```python
from build123d import *

# Parameters (mm, degrees)
SKETCH1_R           = 2.7305
BOSS_EXTRUDE1_DEPTH = 4.6355
SKETCH2_W           = 10.4775
SKETCH2_H           = 9.271
BOSS_EXTRUDE2_DEPTH = 2.54
SKETCH3_W           = 10.4775
SKETCH3_H           = 2.54
SKETCH3_W_2         = 7.8105
SKETCH3_H_2         = 10.4775
BOSS_EXTRUDE3_DEPTH = 7.366
SKETCH4_W           = 3.302
SKETCH4_H           = 6.604
CUT_EXTRUDE1_DEPTH  = 10.4775
FILLET1_R           = 0.762


with BuildPart() as part:
    # Sketch1 → Boss-Extrude1 (new body, symmetric)
    with BuildSketch(Plane(origin=(0, 0, 0), x_dir=(1, 0, 0), z_dir=(0, 1, 0))):
        Polygon((-11.1125, 3.81), (-4.191, 3.81), (-4.191, 9.144), (6.2865, 9.144), (6.2865, -6.6675), (-11.1125, -6.6675), align=None)
        Circle(SKETCH1_R, mode=Mode.SUBTRACT)
    extrude(amount=BOSS_EXTRUDE1_DEPTH, both=True)

    # Sketch2 → Boss-Extrude2 (add)
    with BuildSketch(Plane.ZY.offset(11.1125)):
        with Locations((1.42875, 0)):
            Rectangle(SKETCH2_W, SKETCH2_H)
    extrude(amount=BOSS_EXTRUDE2_DEPTH)

    # Sketch3 → Boss-Extrude3 (add, symmetric)
    with BuildSketch(Plane(origin=(0, 0, 0), x_dir=(1, 0, 0), z_dir=(0, 1, 0))):
        with Locations((1.04775, 7.874)):
            Rectangle(SKETCH3_W, SKETCH3_H)
        with Locations((-9.74725, -1.42875)):
            Rectangle(SKETCH3_W_2, SKETCH3_H_2)
    extrude(amount=BOSS_EXTRUDE3_DEPTH, both=True)

    # Sketch4 → Cut-Extrude1 (cut)
    with BuildSketch(Plane(origin=(0, 0, -3.81), x_dir=(-1, 0, 0), z_dir=(0, 0, -1))):
        with Locations((8.636, 0)):
            Rectangle(SKETCH4_W, SKETCH4_H)
    extrude(amount=-CUT_EXTRUDE1_DEPTH, mode=Mode.SUBTRACT)

    # Fillet1
    fillet1_edges = [part.edges().sort_by_distance(p)[0] for p in [
        (6.2865, 4.6355, 0.03175),
        (-4.191, 0, -3.81),
        (-4.191, 0, -9.144),
        (6.2865, 0, -9.144),
        (6.2865, 0, 6.6675),
        (-5.0165, 4.6355, -3.81),
        (-13.6525, 0, -3.81),
        (-13.6525, 0, 6.6675),
        (-4.191, -4.6355, -5.207),
        (-4.191, 4.6355, -5.207),
        (6.2865, 6.00075, -6.604),
        (-4.191, 6.00075, -6.604),
        (6.2865, -6.00075, -6.604),
        (6.2865, -7.366, -7.874),
        (1.04775, -7.366, -9.144),
        (-4.191, -7.366, -7.874),
        (-4.191, -6.00075, -6.604),
        (1.04775, -7.366, -6.604),
        (6.2865, 7.366, -7.874),
        (1.04775, 7.366, -9.144),
        (-4.191, 7.366, -7.874),
        (1.04775, 7.366, -6.604),
        (0.22225, -4.6355, 6.6675),
        (0.22225, 4.6355, 6.6675),
        (-5.842, 6.00075, 6.6675),
        (-5.842, 6.00075, -3.81),
        (-5.842, -6.00075, 6.6675),
        (-5.842, -7.366, 1.42875),
        (-5.842, -6.00075, -3.81),
        (-9.74725, -7.366, -3.81),
        (-13.6525, -7.366, 1.42875),
        (-9.74725, -7.366, 6.6675),
        (-5.0165, -4.6355, -3.81),
        (-5.842, 7.366, 1.42875),
        (-9.74725, 7.366, -3.81),
        (-13.6525, 7.366, 1.42875),
        (-9.74725, 7.366, 6.6675),
        (6.2865, -4.6355, 0.03175),
    ]]
    fillet(fillet1_edges, radius=FILLET1_R)


solid = part.part
```
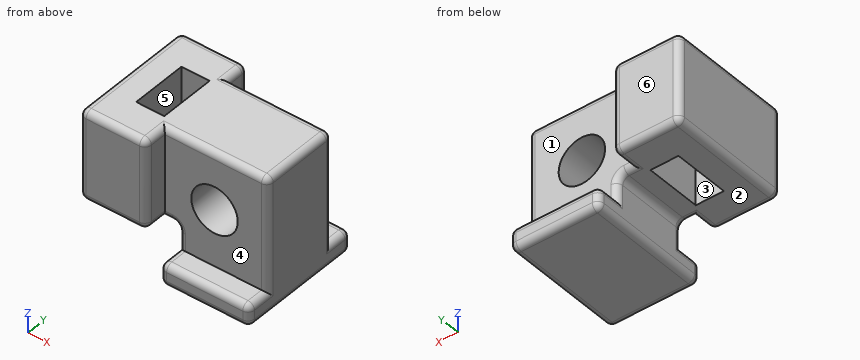
Check sheet for the modelled part. Datum: model origin and axes. Units: mm. Face numbers are marked on the shaded views. A direction names the side the tool comes from. Round coordinates to 2 decimals unless told otherwise and drop trailing zeros. Loops run counter-clockwise (first coordinate to the right, second up) from the corner with the lowest first, then second, coordinate; pieces in that order, holes last. Notation, with made-up numbers: (73, 15.25) -> (94, 15.25) arc R29 ccw to (94, 48.25) -> close; hole circle Ø11 at (74, 74.5). An arc over 180 degrees is marked (long way). Write item = value, one per line. Start each with the question number.
1) Set-up check for the marked faces 1, 2 and 3: record each of +Z, -Z, +X, -X, +Y, -Y from which the full face is reachable in a straight line by a thin tool's end or side.
2) Sectioned sample at C-C, the plane y = -0.25. Record the cut outline in (x, z) (1 decimal), plus the area to 3 significant figures.
3) Sectioned sample at A-A, the plane z = 0. Record the cut outline in (x, y) (1 decimal).
4) Sectioned sample at D-D, the plane x = 0. Record the cut outline in (y, z), plus the area to 3 significant figures.
5) Release check for a two-part mould opening along Y. For the marked faces 4, 5 and 6 record: released by +Y, released by -Y, zero draft, split by the parting line, or undercut.
6) Sectioned sample at B-B, the plane y = 5.25. Record the cut outline in (x, z), plus the area to 3 significant figures.
7) Gauge pin test, flat ends, axial feed: pin 1 Ø6.5 at (x, y) = (-8.5, 0) entering from -Z; pin 2 Ø1.5 at (y, z) = (1, -7) entering from -X; pin 3 Ø2 at (y, z) = (-5, 3) entering from +X. Record the tip position at first contact, or that the pin passes through.
8) Thickness scan on probe 1 along X at (y, z) = (1.75, 0) (1 decimal); probe 2 along Z at (x, y) = (0, -1.5); probe 3 along Y at (x, z) = (-9.75, 2). Record the ranges inside material, lowest first.
Results are:
q1.face_1 = +Z, +X, +Y
q1.face_2 = -Z, -X, +Y, -Y
q1.face_3 = +Z, -Z
q2.outline = (-13.7, -3) arc R0.8 ccw to (-12.9, -3.8) -> (-10.3, -3.8) -> (-10.3, 6.7) -> (-12.9, 6.7) arc R0.8 ccw to (-13.7, 5.9) -> close; (-7, -3.8) -> (-5, -3.8) arc R0.8 cw to (-4.2, -4.6) -> (-4.2, -8.4) arc R0.8 ccw to (-3.4, -9.1) -> (5.5, -9.1) arc R0.8 ccw to (6.3, -8.4) -> (6.3, 5.9) arc R0.8 ccw to (5.5, 6.7) -> (-7, 6.7) -> close; hole circle Ø5.5 at (0, 0)
q2.area = 206 mm^2
q3.outline = (-13.7, -6.6) arc R0.8 ccw to (-12.9, -7.4) -> (-6.6, -7.4) arc R0.8 ccw to (-5.8, -6.6) -> (-5.8, -4.6) -> (-2.7, -4.6) -> (-2.7, 4.6) -> (-5.8, 4.6) -> (-5.8, 6.6) arc R0.8 ccw to (-6.6, 7.4) -> (-12.9, 7.4) arc R0.8 ccw to (-13.7, 6.6) -> close; (2.7, -4.6) -> (5.5, -4.6) arc R0.8 ccw to (6.3, -3.9) -> (6.3, 3.9) arc R0.8 ccw to (5.5, 4.6) -> (2.7, 4.6) -> close; hole (-10.3, -3.3) -> (-7, -3.3) -> (-7, 3.3) -> (-10.3, 3.3) -> close
q4.outline = (-7.37, -8.38) arc R0.76 ccw to (-6.6, -9.14) -> (6.6, -9.14) arc R0.76 ccw to (7.37, -8.38) -> (7.37, -7.37) arc R0.76 ccw to (6.6, -6.6) -> (4.64, -6.6) -> (4.64, -2.73) -> (-4.64, -2.73) -> (-4.64, -6.6) -> (-6.6, -6.6) arc R0.76 ccw to (-7.37, -7.37) -> close; (-4.64, 2.73) -> (4.64, 2.73) -> (4.64, 5.91) arc R0.76 ccw to (3.87, 6.67) -> (-3.87, 6.67) arc R0.76 ccw to (-4.64, 5.91) -> close
q4.area = 109 mm^2
q5.face_4 = released by -Y
q5.face_5 = undercut
q5.face_6 = released by +Y
q6.outline = (-13.65, -3.05) arc R0.76 ccw to (-12.89, -3.81) -> (-6.6, -3.81) arc R0.76 ccw to (-5.84, -3.05) -> (-5.84, 5.91) arc R0.76 ccw to (-6.6, 6.67) -> (-12.89, 6.67) arc R0.76 ccw to (-13.65, 5.91) -> close; (-4.19, -8.38) arc R0.76 ccw to (-3.43, -9.14) -> (5.52, -9.14) arc R0.76 ccw to (6.29, -8.38) -> (6.29, -7.37) arc R0.76 ccw to (5.52, -6.6) -> (-3.43, -6.6) arc R0.76 ccw to (-4.19, -7.37) -> close
q6.area = 107 mm^2
q7.pin_1 = -3.81
q7.pin_2 = -4.19
q7.pin_3 = 6.28
q8.probe_1 = -13.7 to -10.3, -7 to -2.7, 2.7 to 6.3
q8.probe_2 = -9.14 to -2.73, 2.73 to 6.67
q8.probe_3 = -7.37 to -3.3, 3.3 to 7.37
